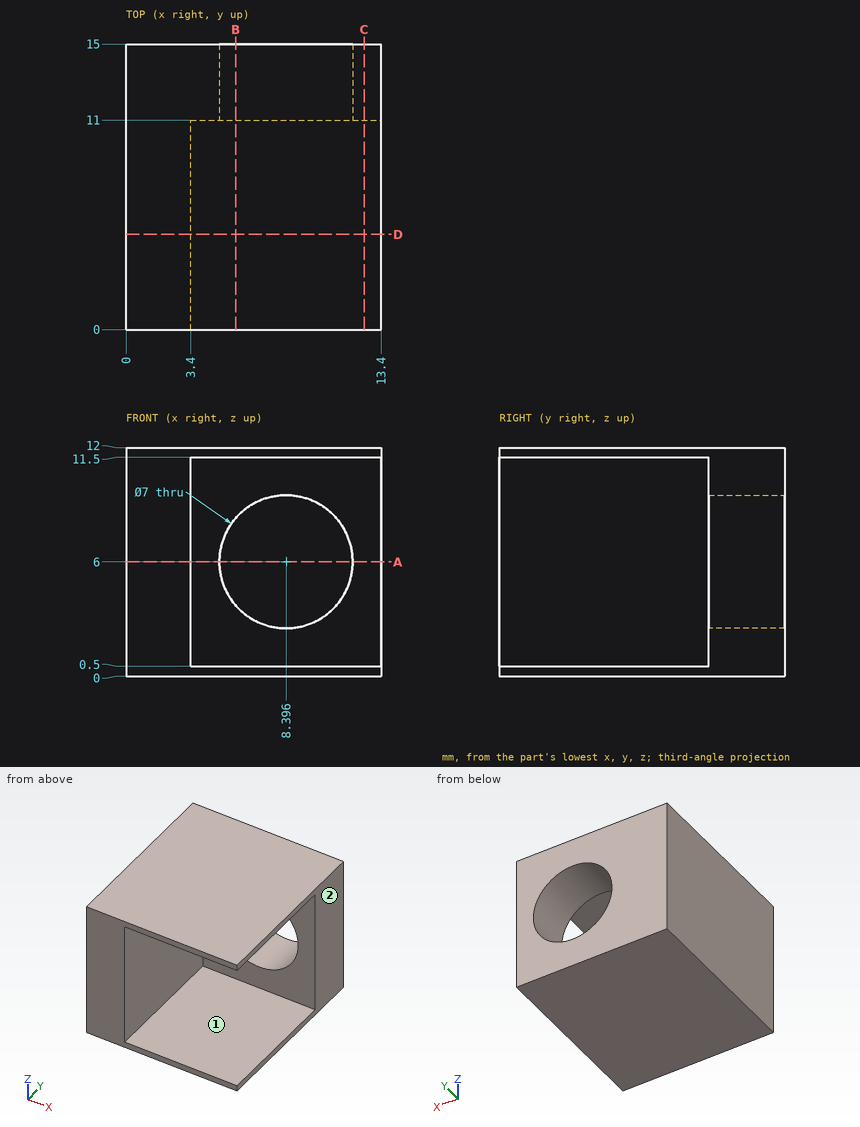
Study the drawing (mm; zero at the part's minimum x, y, z) and answer. A direction names the side the tool comes from. Round coordinates to 2 decimals unless told otherwise and drop trailing zeros. Loops run counter-clockwise (first coordinate to the right, second up) from the corner with the lowest first, then second, coordinate; pieces in that order, holes last. Notation, with made-up numbers: (27, 50) -> (69, 50) arc R24 ccw to (69, 71) -> close; hole circle Ø2 at (-20, -38.5). An arc over 180 degrees is marked (long way). Write each question's results on one line, items separated by ' | '. Start each with the question number.
1. Find the intervals of material crossed by probe 1 along X at (y, z) = (14.15, 6); probe 2 along Z at (x, y) = (10, 9.25); probe 3 along Y at (x, z) = (9.25, 11.25), in increasing order. Write a range as from..to.
2. Section D-D (y = 5) is taken. Determine the outline of the cut face in (x, z).
3. A tool of negligible diameter and unlimited length cuts with its end or side. For the marked faces 1 and 2, from which of +Z, -Z, +X, -X, +Y, -Y can it reach the whole face along a straight path? Write none if from no direction.
4. Section A-A (z = 6) is taken. Determine the outline of the cut face in (x, y), plus the area to 3 significant figures.
5. Section B-B (x = 5.75) is taken. Determine the outline of the cut face in (y, z).
6. Given pin 1 Ø1.5 at (y, z) = (8.5, 7) entering from +X; pin 2 Ø2 at (x, z) = (7.5, 9.5) entering from -Y; pin 3 Ø5.5 at (x, z) = (8.4, 6) entering from -Y, each flat-ended and moving along its own axis, determine where each tip first touches the part or whether it passes through.
7. Section C-C (x = 12.5) is taken. Determine the outline of the cut face in (y, z).
Evaluation:
1) probe 1: x = 0..4.9, 11.9..13.4 | probe 2: z = 0..0.5, 11.5..12 | probe 3: y = 11..15
2) outline: (0, 0) -> (13.4, 0) -> (13.4, 0.5) -> (3.4, 0.5) -> (3.4, 11.5) -> (13.4, 11.5) -> (13.4, 12) -> (0, 12) -> close
3) face 1: +X, -Y | face 2: +Z, -Z, +X, +Y, -Y
4) outline: (0, 0) -> (3.4, 0) -> (3.4, 11) -> (4.9, 11) -> (4.9, 15) -> (0, 15) -> close; (11.9, 11) -> (13.4, 11) -> (13.4, 15) -> (11.9, 15) -> close | area: 63.0 mm2
5) outline: (0, 0) -> (15, 0) -> (15, 3.71) -> (11, 3.71) -> (11, 0.5) -> (0, 0.5) -> close; (0, 11.5) -> (11, 11.5) -> (11, 8.29) -> (15, 8.29) -> (15, 12) -> (0, 12) -> close
6) pin 1: stops at x = 3.4 | pin 2: stops at y = 11 | pin 3: passes through
7) outline: (0, 0) -> (15, 0) -> (15, 12) -> (0, 12) -> (0, 11.5) -> (11, 11.5) -> (11, 0.5) -> (0, 0.5) -> close
